CAD build for the part. Positions are in the model's coordinates, mm. Face numbers are marked on the shaded views. A direction names the side the tool comes from. Round coordinates to 2 decimals unless told otherwise and drop trailing zeros. Loops run counter-clockwise (first coordinate to the right, second up) from the corner with the lowest first, then second, coordinate; pieces in that order, holes last. Notation, with made-up numbers: M 82,-5 L 115,-5 A35 cw 115,28 Z; hole C 66.5,11.25 d5. An arc over 180 degrees is marked long. One line per item, written item: value. Start each with the question number.
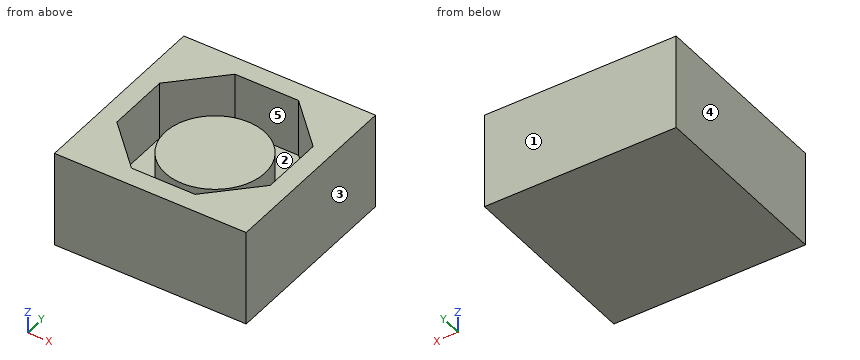
from build123d import *

# Parameters (mm, degrees)
F0_W     = 10
F0_H     = 10
F1_DEPTH = 5
F3_DEPTH = 3
F4_R     = 2.6
F5_DEPTH = 2


with BuildPart() as f1:
    # F0 (on Top) → F1 (new body)
    with BuildSketch(Plane.XY):
        Rectangle(F0_W, F0_H)
    extrude(amount=F1_DEPTH)

    # F2 (on face) → F3 (cut)
    with BuildSketch(Plane.XY.offset(5)):
        Polygon((-4, 1.656854), (-4, -1.656854), (-1.656854, -4), (1.656854, -4), (4, -1.656854), (4, 1.656854), (1.656854, 4), (-1.656854, 4), align=None)
    extrude(amount=-F3_DEPTH, mode=Mode.SUBTRACT)

    # F4 (on face) → F5 (join)
    with BuildSketch(Plane.XY.offset(2)):
        Circle(F4_R)
    extrude(amount=F5_DEPTH)


solid = f1.part
(1) Mould opens along X. For the marked faces 1, 2 and 3 say: pulls with the +X half, pulls with the -X half, needs draft (parallel to the pull), parting line crosses it, or undercut.
(2) Slice it at D-D, the plane z = 4.75. List the corners of the cut face in (x, y), and give its area (3 significant figures).
(3) Flat gauge pins, fed straight in: P1, Ø4, axis at x = -1, y = -2, coming from the +Z side; P2, Ø5.5, axis at x = -0.5, y = 0, coming from the +Z side. Where does each tip first touch, or does it go through?
(4) Slice it at A-A, the plane z = 3.4. List the corners of the cut face in (x, y), and give its area (3 significant figures).
(5) Probe L1, parallel to X at y = 1.5, z = 4.1; L2, parallel to Y at x = 0, z = 2.3. List the from-to ranges inside material, lowest first.
(6) Which spindle directions (+Z, -Z, +X, -X, +Y, -Y) get a long thin tool onto all of the face, cutting with end or side? Do the marked faces 4 and 5. Say none if no direction does.
(7) Slice it at B-B, the plane y = 0. List the corners of the cut face in (x, z).
Check result:
1. face 1: needs draft
1. face 2: undercut
1. face 3: pulls with the +X half
2. outline: M -5,-5 L 5,-5 L 5,5 L -5,5 Z; hole M -4,-1.66 L -1.66,-4 L 1.66,-4 L 4,-1.66 L 4,1.66 L 1.66,4 L -1.66,4 L -4,1.66 Z
2. area: 47.0 mm^2
3. P1: stops at z = 5
3. P2: stops at z = 4
4. outline: M -5,-5 L 5,-5 L 5,5 L -5,5 Z; C 0,0 d5.2; hole M -4,-1.66 L -1.66,-4 L 1.66,-4 L 4,-1.66 L 4,1.66 L 1.66,4 L -1.66,4 L -4,1.66 Z
4. area: 68.2 mm^2
5. L1: x = -5 to -4, 4 to 5
5. L2: y = -5 to -4, -2.6 to 2.6, 4 to 5
6. face 4: +Z, -Z, -X, +Y, -Y
6. face 5: +Z
7. outline: M -5,0 L 5,0 L 5,5 L 4,5 L 4,2 L 2.6,2 L 2.6,4 L -2.6,4 L -2.6,2 L -4,2 L -4,5 L -5,5 Z
